Can you work these out from the model? Positions are in its coordinate system, mm. Face numbers are marked on the shaded views. A direction names the side the tool comes from. Round coordinates to 2 decimals unless told otherwise and drop trailing zeros. Write each loop counter-clockwise with the first axis right and the second up, starting at its lowest first coordinate (ties: lowest second). Pieces come first, ordered by that corner, then holes.
Q1. Please list where these lines run through material, in increasing order: line 1 along Z through (x, y) = (-1.5, 4.65); line 2 along X through (y, z) = (2, 99); line 3 along X through (y, z) = (-1, 28).
Q2. I'm going to push flat-ended pins straight in: pin 1 Ø10 at (x, y) = (-5.5, -21) entering from +Z; pin 2 Ø2 at (x, z) = (25.5, 34.5) entering from +Y; pin 3 Ø2 at (x, y) = (-16, -22.5) entering from -Z; pin 4 Ø3.5 at (x, z) = (-1.5, 28) entering from +Y. Where does each tip first touch, or does it pass through?
Q3. If we section it at C-C (z = 129): Please give me the cut outline in (x, y).
Q4. For the marked faces 1, 2, 3, 4 and 5, which set-ups out of +Z, -Z, +X, -X, +Y, -Y let a thin tool reach every point of the face, with its end or its side?
Q5. If we section it at D-D (z = 94.5): Please give me the cut outline in (x, y).
Q6. If we section it at A-A (z = 28): Give the number of separate pieces and of enclosed holes in the cut face, plus the area to 3 significant figures.
Q7. If we section it at B-B (x = 25.5): Please give me the cut outline in (y, z).
Q8. We'd pull the mould along Z, two halves only. Please class the marked faces 6, 7, 8 and 9: +Z half, -Z half, draft (parallel to the pull), parting line (faces both ways), or undercut.
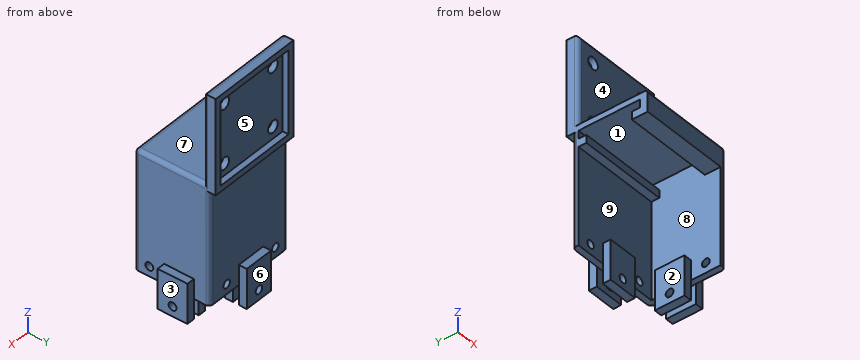
Autodesk Inventor part; units mm, degrees
ref_plane "YZ Plane" through (0, 0, 0) normal (1, 0, 0) x (0, 1, 0)
ref_plane "XZ Plane" through (0, 0, 0) normal (0, 1, 0) x (-1, 0, 0)
ref_plane "XY Plane" through (0, 0, 0) normal (0, 0, 1) x (1, 0, 0)
sketch "Sketch1" plane through (0, 0, 0) normal (0, 1, 0) x (-1, 0, 0)
  line L0 (24, 138) -> (-24, 138)
  line L1 (-24, 138) -> (-24, -138)
  line L2 (-24, -138) -> (24, -138)
  line L3 (24, -138) -> (24, 138)
  point P0 (0, 0)
  dimension "d0" = 48
  dimension "d1" = 276
extrude "Extrusion1" add sketch "Sketch1" along normal blind 3
sketch "Sketch2" plane through (0, 3, 0) normal (0, 1, 0) x (1, 0, 0)
  line L0 (-24, 138) -> (-24, -138)
  line L1 (-24, -138) -> (-21, -138)
  line L2 (-21, -138) -> (-21, -90)
  line L3 (-21, -90) -> (-24, -90)
  line L4 (-24, -90) -> (-24, -138)
  line L5 (24, -138) -> (24, 138)
  line L6 (-21, -90) -> (24, -90)
  line L7 (24, -90) -> (24, -93)
  line L8 (24, -93) -> (-21, -93)
  line L9 (-21, -93) -> (-21, -90)
  line L10 (-24, -138) -> (24, -138)
  line L11 (24, -93) -> (21, -93)
  line L12 (21, -93) -> (21, -138)
  line L13 (21, -138) -> (24, -138)
  line L14 (24, -138) -> (24, -93)
  line L15 (21, -138) -> (-21, -138)
  line L16 (-21, -138) -> (-21, -135)
  line L17 (-21, -135) -> (21, -135)
  line L18 (21, -135) -> (21, -138)
  point P0 (0, 0)
  dimension "d4" = 3
  dimension "d5" = 48
  dimension "d6" = 3
  dimension "d7" = 3
  dimension "d8" = 3
extrude "Extrusion2" add sketch "Sketch2" along normal blind 3 contours L3 L2 L1 L0 | L6 L5 L8 L2 | L2 L17 L12 L10 | L12 L8 L5 L10
mirror "Mirror1" about plane through (0, 0, 0) normal (0, 0, 1) of "Extrusion2"
sketch "Sketch3" plane through (0, 0, 0) normal (0, -1, 0) x (1, 0, 0)
  line L0 (24, -90) -> (-24, -90)
  line L1 (24, 138) -> (24, -138)
  line L2 (-24, -90) -> (24, -90)
  line L3 (24, -90) -> (24, -93)
  line L4 (24, -93) -> (-24, -93)
  line L5 (-24, -93) -> (-24, -90)
  line L6 (-24, 90) -> (24, 90)
  line L7 (24, 90) -> (21, 90)
  line L8 (21, 90) -> (21, -90)
  line L9 (21, -90) -> (24, -90)
  line L10 (24, -90) -> (24, 90)
  line L11 (-24, 90) -> (24, 90)
  line L12 (24, 90) -> (24, 93)
  line L13 (24, 93) -> (-24, 93)
  line L14 (-24, 93) -> (-24, 90)
  point P0 (0, 0)
  dimension "d11" = 3
  dimension "d12" = 3
  dimension "d13" = 3
extrude "Extrusion3" add sketch "Sketch3" along normal blind 35
sketch "Sketch4" plane through (-24, 0, -90) normal (0, 0, 1) x (1, 0, 0)
  line L0 (0, -35) -> (45, -35)
  line L1 (45, 0) -> (45, -35)
  line L2 (0, -35) -> (45, -35)
  line L3 (45, -35) -> (45, -31)
  line L4 (45, -31) -> (0, -31)
  line L5 (0, -31) -> (0, -35)
  point P0 (24, 0)
  dimension "d16" = 4
extrude "Extrusion4" add sketch "Sketch4" along normal blind 8
sketch "Sketch5" plane through (-24, -31, -90) normal (0, 1, 0) x (1, 0, 0)
  line L0 (0, -8) -> (45, -8)
  line L1 (45, 0) -> (45, -8)
  line L2 (0, -8) -> (45, -8)
  line L3 (45, -8) -> (45, -4)
  line L4 (45, -4) -> (0, -4)
  line L5 (0, -4) -> (0, -8)
  point P0 (24, -90)
  dimension "d19" = 4
extrude "Extrusion5" add sketch "Sketch5" along normal blind 4
sketch "Sketch6" plane through (0, 0, 0) normal (0, -1, 0) x (1, 0, 0)
  line L0 (21, -86) -> (-24, -86)
  line L1 (-24, -82) -> (21, -82)
  line L2 (21, -82) -> (21, -86)
  line L3 (21, -86) -> (-24, -86)
  line L4 (-24, -86) -> (-24, -82)
  point P0 (0, 0)
  dimension "d22" = 4
extrude "Extrusion6" add sketch "Sketch6" along normal blind 4
mirror "Mirror2" about plane through (0, 0, 0) normal (0, 0, 1) of "Extrusion6", "Extrusion5", "Extrusion4"
sketch "Sketch7" plane through (0, 0, 0) normal (0, -1, 0) x (1, 0, 0)
  circle A0 centre (-15, -129) radius 3
  circle A1 centre (15, -129) radius 3
  circle A2 centre (15, -99) radius 3
  circle A3 centre (-15, -99) radius 3
  point P0 (0, 0)
  dimension "d25" = 6
  dimension "d26" = 6
  dimension "d27" = 6
  dimension "d28" = 6
extrude "Extrusion7" cut sketch "Sketch7" against normal blind 4
mirror "Mirror3" about plane through (0, 0, 0) normal (0, 0, 1) of "Extrusion7"
sketch "Sketch8" plane through (0, 0, 0) normal (0, -1, 0) x (1, 0, 0)
  line L0 (21, 82) -> (21, -82)
  line L1 (-24, -82) -> (-24, 82)
  line L2 (21, -20) -> (-24, -20)
  line L3 (-24, -20) -> (-24, -17)
  line L4 (-24, -17) -> (21, -17)
  line L5 (21, -17) -> (21, -20)
  point P0 (0, 0)
  dimension "d31" = 3
extrude "Extrusion8" add sketch "Sketch8" along normal blind 42.3
sketch "Sketch9" plane through (21, 0, -20) normal (0, 0, -1) x (-1, 0, 0)
  circle A0 centre (39.35, -5.65) radius 4
  circle A1 centre (39.35, -36.65) radius 4
  circle A2 centre (8.35, -5.65) radius 4
  circle A3 centre (8.35, -36.65) radius 4
  point P0 (21, 0)
  dimension "d34" = 8
  dimension "d35" = 8
  dimension "d36" = 8
  dimension "d37" = 8
extrude "Extrusion9" add sketch "Sketch9" along normal blind 3
sketch "Sketch10" plane through (-18.35, -36.65, -23) normal (0, 0, -1) x (-1, 0, 0)
  circle A0 centre (0, 0) radius 3
  circle A1 centre (0, 31) radius 4
  circle A2 centre (0, 31) radius 3
  circle A3 centre (-31, 0) radius 4
  circle A4 centre (-31, 0) radius 3
  circle A5 centre (-31, 31) radius 4
  circle A6 centre (-31, 31) radius 3
  point P0 (-18.35, 36.65)
  dimension "d40" = 6
  dimension "d41" = 6
  dimension "d42" = 6
  dimension "d43" = 6
extrude "Extrusion10" cut sketch "Sketch10" against normal blind 2 contours A0 | A2 | A4 | A6
sketch "Sketch11" plane through (21, 0, -20) normal (0, 0, -1) x (-1, 0, 0)
  circle A0 centre (23.85, -21.15) radius 12.5
  circle A1 centre (39.35, -36.65) radius 3
  circle A2 centre (39.35, -36.65) radius 2
  circle A3 centre (8.35, -36.65) radius 3
  circle A4 centre (8.35, -36.65) radius 2
  circle A5 centre (8.35, -5.65) radius 4
  circle A6 centre (8.35, -5.65) radius 2
  circle A7 centre (39.35, -5.65) radius 4
  circle A8 centre (39.35, -5.65) radius 2
  point P0 (21, 0)
  dimension "d46" = 25
  dimension "d47" = 4
  dimension "d48" = 4
  dimension "d49" = 4
  dimension "d50" = 4
extrude "Extrusion11" cut sketch "Sketch11" along normal mid plane 10 contours A0 | A2 | A4 | A6 | A8
sketch "Sketch12" plane through (0, 0, 0) normal (0, -1, 0) x (1, 0, 0)
  line L0 (-24, -17) -> (-24, 82)
  line L1 (-24, 33) -> (24, 33)
  line L2 (24, 33) -> (24, -138)
  line L3 (24, -138) -> (-24, -138)
  line L4 (-24, -138) -> (-24, 33)
  point P0 (0, 0)
extrude "Extrusion12" cut sketch "Sketch12" along normal mid plane 100
sketch "Sketch13" plane through (0, 0, 0) normal (0, -1, 0) x (1, 0, 0)
  line L0 (-9, 43) -> (6, 43)
  line L1 (6, 43) -> (6, 23)
  line L2 (6, 23) -> (-9, 23)
  line L3 (-9, 23) -> (-9, 43)
  point P0 (0, 0)
  dimension "d55" = 15
  dimension "d56" = 20
extrude "Extrusion13" add sketch "Sketch13" along normal blind 4 and the other way blind 7
sketch "Sketch14" plane through (21, 0, 86) normal (-1, 0, 0) x (0, 0, 1)
  line L0 (-43, -20) -> (-63, -20)
  line L1 (-63, -20) -> (-63, -5)
  line L2 (-63, -5) -> (-43, -5)
  line L3 (-43, -5) -> (-43, -20)
  point P0 (-86, 0)
  dimension "d61" = 20
  dimension "d62" = 15
extrude "Extrusion14" add sketch "Sketch14" along normal blind 4 and the other way blind 7
sketch "Sketch15" plane through (21, 0, 86) normal (-1, 0, 0) x (0, 0, 1)
  circle A0 centre (-58, -12.5) radius 2
  circle A1 centre (-48, -27.5) radius 2
  point P0 (-86, 0)
  dimension "d67" = 4
  dimension "d68" = 4
extrude "Extrusion15" cut sketch "Sketch15" along normal mid plane 20
sketch "Sketch16" plane through (0, 0, 0) normal (0, -1, 0) x (1, 0, 0)
  circle A0 centre (-16.5, 38) radius 2
  circle A1 centre (-1.5, 28) radius 2
  circle A2 centre (13.5, 38) radius 2
  point P0 (0, 0)
  dimension "d71" = 4
  dimension "d72" = 4
  dimension "d73" = 4
extrude "Extrusion16" cut sketch "Sketch16" along normal mid plane 20
sketch "Sketch17" plane through (6, -4, 23) normal (0, 0, -1) x (-1, 0, 0)
  line L0 (-18, 7) -> (0, 7)
  line L1 (15, 4) -> (15, 0)
  line L2 (0, 7) -> (15, 7)
  line L3 (15, 7) -> (15, 4)
  line L4 (15, 4) -> (0, 4)
  line L5 (0, 4) -> (0, 7)
  line L6 (-15, -16) -> (-18, -16)
  line L7 (-18, -16) -> (-18, -1)
  line L8 (-18, -1) -> (-15, -1)
  line L9 (-15, -1) -> (-15, -16)
  point P0 (6, 4)
  dimension "d76" = 3
extrude "Extrusion17" cut sketch "Sketch17" against normal blind 10
fillet "Fillet1" radius 2 8 edges at (-24, 0, 115.5) (0, 0, 138) (24, 0, 115.5) (0, -35, 93) (-24, 3, 61.5) (24, -35, 63) (24, 3, 61.5) (24, -17.5, 93)
properties part number "carriageEndR"
A:
1. line 1: z = 23 to 26, 30 to 43, 90 to 93, 135 to 138
1. line 2: x = -24 to -18, -12 to 12, 18 to 24
1. line 3: x = -9 to -3.5, 0.5 to 6
2. pin 1: stops at z = 93
2. pin 2: stops at y = -5
2. pin 3: stops at z = 90
2. pin 4: passes through
3. outline: (-24, 2) arc R2 ccw to (-22, 0) - (-18, 0) - (-18, 3) - (-21, 3) - (-21, 6) - (-24, 6) - close; (-12, 0) - (12, 0) - (12, 3) - (-12, 3) - close; (18, 0) - (22, 0) arc R2 ccw to (24, 2) - (24, 6) - (21, 6) - (21, 3) - (18, 3) - close
4. face 1: -X
4. face 2: -Z, -X, -Y
4. face 3: +Z, -Z, +X, +Y, -Y
4. face 4: +Z, +X, -X, -Y
4. face 5: +Y
5. outline: (-24, 2) arc R2 ccw to (-22, 0) - (22, 0) arc R2 ccw to (24, 2) - (24, 6) - (21, 6) - (21, 3) - (-21, 3) - (-21, 6) - (-24, 6) - close
6. separate pieces: 8
6. enclosed holes: 0
6. area: 176 mm2
7. outline: (-20, 23) - (-5, 23) - (-5, 43) - (-20, 43) - close; hole circle Ø4 at (-12.5, 28)
8. face 6: draft
8. face 7: +Z half
8. face 8: undercut
8. face 9: undercut
